Part model, mm, in its own coordinate system. A direction names the side the tool comes from. Coordinates: 2 decimals unless noted, no trailing zeros. Order: outer loops, then holes, each group sorted by start corner. A loop starts at its lowest first (then second) coordinate and runs counter-clockwise, first axis right, second up.
from build123d import *

# Parameters (mm, degrees)
SKETCH1_W            = 43.5
SKETCH1_H            = 39.5
BODY_DEPTH           = 1
SKETCH2_W            = 1
SKETCH2_H            = 3
CLIPS_R_DEPTH        = 2
SKETCH3_W            = 1
SKETCH3_H            = 3
CLIPS_L_DEPTH        = 2
SKETCH4_W            = 8.299556423
SKETCH4_H            = 1
CLIPS_B_DEPTH        = 2
SKETCH5_R            = 3.375
PADDLE_SUPPORT_DEPTH = 3
SKETCH6_R            = 2.875
BOLTS_DEPTH          = 5
FILLET1_R            = 3


with BuildPart() as part:
    # Sketch1 → body (new body)
    with BuildSketch(Plane.XY):
        Rectangle(SKETCH1_W, SKETCH1_H)
    extrude(amount=BODY_DEPTH)

    # Sketch2 → clips_r (add)
    with BuildSketch(Plane(origin=(21.75, 0, 0), x_dir=(0, 0, -1), z_dir=(1, 0, 0))):
        with Locations((-0.5, 16.25)):
            Rectangle(SKETCH2_W, SKETCH2_H)
        with Locations((-0.5, -13.25)):
            Rectangle(SKETCH2_W, SKETCH2_H)
    extrude(amount=CLIPS_R_DEPTH)

    # Sketch3 → clips_l (add)
    with BuildSketch(Plane.ZY.offset(21.75)):
        with Locations((0.5, -13.25)):
            Rectangle(SKETCH3_W, SKETCH3_H)
        with Locations((0.5, 16.25)):
            Rectangle(SKETCH3_W, SKETCH3_H)
    extrude(amount=CLIPS_L_DEPTH)

    # Sketch4 → clips_b (add)
    with BuildSketch(Plane.XZ.offset(19.75)):
        with Locations((0.100221788, 0.5)):
            Rectangle(SKETCH4_W, SKETCH4_H)
    extrude(amount=CLIPS_B_DEPTH)

    # Sketch5 → paddle_support (add)
    with BuildSketch(Plane.XY.offset(1)):
        with Locations((9.250464542, -11.75)):
            Circle(SKETCH5_R)
        with Locations((-9.250464542, -11.75)):
            Circle(SKETCH5_R)
    extrude(amount=PADDLE_SUPPORT_DEPTH)

    # Sketch6 → bolts (cut, through all)
    with BuildSketch(Plane.XY.offset(4)):
        with Locations((-9.250464542, -11.75)):
            Circle(SKETCH6_R)
        with Locations((9.250464542, -11.75)):
            Circle(SKETCH6_R)
    extrude(amount=-BOLTS_DEPTH, mode=Mode.SUBTRACT)

    # Fillet1
    fillet1_edges = [part.edges().sort_by_distance(p)[0] for p in [
        (21.75, -19.75, 0.5),
        (-21.75, -19.75, 0.5),
    ]]
    fillet(fillet1_edges, radius=FILLET1_R)


solid = part.part
Q1. Wall check: line 1 along Y through (x, z) = (-9, 0.9); line 2 along X through (y, z) = (-16, 0.75); line 3 along Z through (x, y) = (-11, 15.5). Give the ranges that are in metal, low to high.
Results list:
line 1: y = -19.75 to -14.61, -8.89 to 19.75
line 2: x = -21.75 to 21.75
line 3: z = 0 to 1
Q2. Mould opens along Y. For faces 1 (the face through (21.75, 18.7, 0.5)), 2 (the face through (-11.5, -19.75, 0.5)), 3 (the face through (-22.7, -11.75, 0.5)) say: pulls with the +Y half, pulls with the -Y half, needs draft (parallel to the pull), parting line crosses it, or undercut.
Results list:
face 1: needs draft
face 2: pulls with the -Y half
face 3: undercut
Q3. Cut at D-D on x = -16. Write the cut outline in (y, z), and give its area (3 significant figures).
Results list:
outline: (-19.75, 0) - (19.75, 0) - (19.75, 1) - (-19.75, 1) - close
area: 39.5 mm2
Q4. Which spindle directions (+Z, -Z, +X, -X, +Y, -Y) get a long thin tool onto all of the face, cutting with end or side? Do faces 4 (the face through (-21.75, 1.3, 0.5)), 5 (the face through (22.7, 14.75, 0.5)), 6 (the face through (-22.7, -14.75, 0.5)), 7 (the face through (4.25, -20.7, 0.5)), 8 (the face through (-0.3, 19.75, 0.5)). Say none if no direction does.
Results list:
face 4: +Z, -Z, -X
face 5: +Z, -Z, +X
face 6: +Z, -Z, -X, -Y
face 7: +Z, -Z, +X, -Y
face 8: +Z, -Z, +X, -X, +Y
Q5. Pin check, flat tips, straight feed: pin 1 Ø8 at (x, y) = (11.5, 0) entering from +Z; pin 2 Ø0.5 at (x, z) = (-23, 0.5) entering from +Y; pin 3 Ø1.1 at (x, z) = (-10.5, 0.5) entering from -Y; pin 4 Ø1.5 at (y, z) = (-3.5, 2) entering from -X. Stop position of each tip, or through.
Results list:
pin 1: stops at z = 1
pin 2: stops at y = 17.75
pin 3: stops at y = -19.75
pin 4: passes through
Q6. Cut at A-A on y = -13. Write the cut outline in (x, z).
Results list:
outline: (-23.75, 0) - (-11.84, 0) - (-11.84, 4) - (-12.39, 4) - (-12.39, 1) - (-23.75, 1) - close; (-6.66, 0) - (6.66, 0) - (6.66, 4) - (6.12, 4) - (6.12, 1) - (-6.12, 1) - (-6.12, 4) - (-6.66, 4) - close; (11.84, 0) - (23.75, 0) - (23.75, 1) - (12.39, 1) - (12.39, 4) - (11.84, 4) - close
Q7. Cut at B-B on z = 2.45. Write the cut outline in (x, y) (3 decimals), and give its area (3 significant figures).
Results list:
outline: circle Ø6.75 at (-9.25, -11.75); circle Ø6.75 at (9.25, -11.75); hole circle Ø5.75 at (-9.25, -11.75); hole circle Ø5.75 at (9.25, -11.75)
area: 19.6 mm2
Q8. Cut at C-C on y = 12.5. Write the cut outline in (x, z), and give its area (3 significant figures).
Results list:
outline: (-21.75, 0) - (21.75, 0) - (21.75, 1) - (-21.75, 1) - close
area: 43.5 mm2
